Part model, mm, in its own coordinate system. A direction names the side the tool comes from. Give positions to 0.01 mm unless a question says otherwise; leave off trailing zeros. Order: outer loops, then holes, each group sorted by start corner. A loop starts at its lowest first (then second) coordinate and runs counter-clockwise, first axis right, second up.
from build123d import *

# Parameters (mm, degrees)
SKETCH1_W           = 12
SKETCH1_H           = 18.3
BOSS_EXTRUDE1_DEPTH = 3
SKETCH2_W           = 6
SKETCH2_H           = 8.7
BOSS_EXTRUDE2_DEPTH = 6
SKETCH3_R           = 1.575
CUT_EXTRUDE1_DEPTH  = 22.257704486
FILLET1_R           = 3
SKETCH4_W           = 6
SKETCH4_H           = 8.7
BOSS_EXTRUDE3_DEPTH = 3
SKETCH5_W           = 6
SKETCH5_H           = 18.3
CUT_EXTRUDE2_DEPTH  = 3
FILLET2_R           = 3
BOSS_EXTRUDE4_DEPTH = 6


with BuildPart() as part:
    # Sketch1 → Boss-Extrude1 (new body)
    with BuildSketch(Plane(origin=(0, 0, 0), x_dir=(1, 0, 0), z_dir=(0, 1, 0))):
        Rectangle(SKETCH1_W, SKETCH1_H)
    extrude(amount=BOSS_EXTRUDE1_DEPTH)

    # Sketch2 → Boss-Extrude2 (add)
    with BuildSketch(Plane(origin=(0, 3, 0), x_dir=(1, 0, 0), z_dir=(0, 1, 0))):
        with Locations((-3, 0)):
            Rectangle(SKETCH2_W, SKETCH2_H)
    extrude(amount=BOSS_EXTRUDE2_DEPTH)

    # Sketch3 → Cut-Extrude1 (cut, through all)
    with BuildSketch(Plane.XY.offset(9.15)):
        with Locations((-3, 6)):
            Circle(SKETCH3_R)
    extrude(amount=-CUT_EXTRUDE1_DEPTH, mode=Mode.SUBTRACT)

    # Fillet1
    fillet1_edges = [part.edges().sort_by_distance(p)[0] for p in [
        (-6, 9, 0),
        (0, 9, 0),
    ]]
    fillet(fillet1_edges, radius=FILLET1_R - 0.0001)  # a hair under: the kernel refuses the full size

    # Sketch4 → Boss-Extrude3 (add)
    with BuildSketch(Plane(origin=(0, 3, 0), x_dir=(1, 0, 0), z_dir=(0, 1, 0))):
        with Locations((3, 0)):
            Rectangle(SKETCH4_W, SKETCH4_H)
    extrude(amount=BOSS_EXTRUDE3_DEPTH)

    # Sketch5 → Cut-Extrude2 (cut)
    with BuildSketch(Plane.XZ):
        with Locations((-3, 0)):
            Rectangle(SKETCH5_W, SKETCH5_H)
    extrude(amount=-CUT_EXTRUDE2_DEPTH, mode=Mode.SUBTRACT)

    # Fillet2
    fillet2_edges = [part.edges().sort_by_distance(p)[0] for p in [
        (-6, 3, 0),
    ]]
    fillet(fillet2_edges, radius=FILLET2_R)

    # Sketch6 → Boss-Extrude4 (add)
    with BuildSketch(Plane(origin=(6, 0, 0), x_dir=(0, 0, -1), z_dir=(1, 0, 0))):
        Polygon((4.35, 3), (6.75, 3), (4.35, 6), align=None)
        Polygon((-4.35, 3), (-4.35, 6), (-6.75, 3), align=None)
    extrude(amount=-BOSS_EXTRUDE4_DEPTH)


solid = part.part
Item 1: Drill centre lines: probe 1 along Y at (x, z) = (-3, 1.5) (3 decimals); probe 2 along Z at (x, y) = (-0.25, 3.75); probe 3 along X at (y, z) = (1.25, 5.25). Where is each one in solid material? Low to high.
Item 2: Band-saw the part on D-D on y = 1. List the corners of the cut face in (x, z).
Item 3: Which spindle directions (+Z, -Z, +X, -X, +Y, -Y) get a long thin tool onto all of the face, cutting with end or side? Do faces 1 (the face through (-1.7, 4.6, 4.35)), 2 (the face through (3, 3, -8)), 3 (the face through (3, 3, 8)), 4 (the face through (-1.7, 4.6, -4.35)). Say none if no direction does.
Item 4: Band-saw the part on B-B on x = 1.25. List the corners of the cut face in (y, z).
Item 5: Band-saw the part on C-C on x = -3.25. List the corners of the cut face in (y, z).
Item 6: Drop flat-ended pins along their axis: P1, Ø0.7, axis at x = 2, z = -8.5, coming from the +Y side; P2, Ø2, axis at x = -1, y = 6.5, coming from the -Z side; P3, Ø3, axis at y = 2, z = 1.5, coming from the -X side. Give the stop position or say it passes through.
Working result:
1. probe 1: y = 3 to 4.425, 7.575 to 9
1. probe 2: z = -4.35 to 4.35
1. probe 3: x = 0 to 6
2. outline: (0, -9.15) - (6, -9.15) - (6, 9.15) - (0, 9.15) - close
3. face 1: +Z, -X, +Y, -Y
3. face 2: -Z, +X, -X, +Y
3. face 3: +Z, +X, -X, +Y
3. face 4: -Z, -X, +Y, -Y
4. outline: (0, -9.15) - (3, -9.15) - (3, -6.75) - (6, -4.35) - (6, 4.35) - (3, 6.75) - (3, 9.15) - (0, 9.15) - close
5. outline: (3.01, -4.35) - (4.44, -4.35) - (4.44, 4.35) - (3.01, 4.35) - close; (7.56, -4.35) - (8.99, -4.35) - (8.99, 4.35) - (7.56, 4.35) - close
6. P1: stops at y = 3
6. P2: stops at z = -4.35
6. P3: stops at x = -4.66
